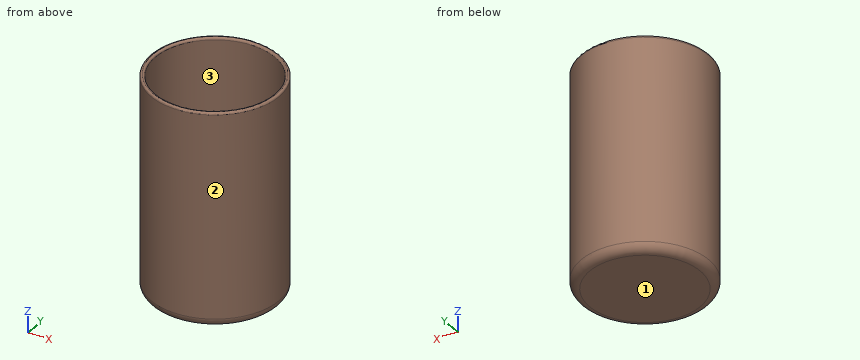
```python
from build123d import *

# Parameters (mm, degrees)
F0_R     = 38.1
F0_R_2   = 35.56
F1_DEPTH = 127
F2_R     = 38.1
F3_DEPTH = 25.4
F4_R     = 1.26999
F5_R     = 5.08
F6_R     = 5.08


# Not quite as in the source:
# - a fillet or chamfer is up to 0.001 mm smaller than in the source, because OpenCascade refuses the exact size


with BuildPart() as f1:
    # F0 (on Top) → F1 (new body)
    with BuildSketch(Plane.XY):
        Circle(F0_R)
        Circle(F0_R_2, mode=Mode.SUBTRACT)
    extrude(amount=F1_DEPTH)

    # F2 (on Top) → F3 (join)
    with BuildSketch(Plane.XY):
        Circle(F2_R)
    extrude(amount=F3_DEPTH)

    # F4 (radius 1.27 in the source; OpenCascade refuses exactly that, so slightly less here)
    f4_edges = [f1.edges().sort_by_distance(p)[0] for p in [
        (-38.1, 0, 127),
        (-35.56, 0, 127),
    ]]
    fillet(f4_edges, radius=F4_R)

    # F5
    f5_edges = [f1.edges().sort_by_distance(p)[0] for p in [
        (-38.1, 0, 0),
    ]]
    fillet(f5_edges, radius=F5_R)

    # F6
    f6_edges = [f1.edges().sort_by_distance(p)[0] for p in [
        (-35.56, 0, 25.4),
    ]]
    fillet(f6_edges, radius=F6_R)


solid = f1.part
```
Could you check a few things on this model? Use its own coordinates, in mm. Face numbers are marked on the shaded views. Coordinates: 2 decimals unless noted, no trailing zeros. Write each loop counter-clockwise with the first axis right and the second up, starting at its lowest first coordinate (ties: lowest second). Pieces come first, ordered by that corner, then holes. Notation, with made-up numbers: (-3.75, 37.25) - (30.25, 37.25) arc R12 ccw to (30.25, 56.25) - close; hole circle Ø10 at (60, 61). An arc over 180 degrees is marked (long way). Use a Markdown table: item, result.
Q1. Please list where these lines run through material, in increasing order: L1, parallel to Y at x = 0, z = 65; L2, parallel to Z at x = 1, y = 15; L3, parallel to Y at x = 30.5, z = 77.5.
Geometry check:
| item | result |
|---|---|
| L1 | y = -38.1 to -35.56, 35.56 to 38.1 |
| L2 | z = 0 to 25.4 |
| L3 | y = -22.83 to -18.28, 18.28 to 22.83 |
Q2. Thinking about a two-plate mould opening in X: for the marked faces 1, 2 and 3, which applies, +X half, -X half, draft (parallel to the pull), parting line (faces both ways), or undercut?
Geometry check:
| item | result |
|---|---|
| face 1 | draft |
| face 2 | parting line |
| face 3 | undercut |
Q3. Imagine slicing it at D-D (z = 16). List the corners of the cut face in (x, y) for me.
Geometry check:
| item | result |
|---|---|
| outline | circle Ø76.2 at (0, 0) |
Q4. I'm going to push flat-ended pins straight in: pin 1 Ø1 at (x, z) = (15, 64) entering from -Y; pin 2 Ø12 at (x, z) = (0, 80) entering from -Y; pin 3 Ø1 at (x, z) = (-10.5, 86) entering from +Y. Where does each tip first touch, or does it pass through?
Geometry check:
| item | result |
|---|---|
| pin 1 | stops at y = -35.23 |
| pin 2 | stops at y = -38.1 |
| pin 3 | stops at y = 36.76 |
Q5. Imagine slicing it at C-C (z = 66). List the corners of the cut face in (x, y) for me.
Geometry check:
| item | result |
|---|---|
| outline | circle Ø76.2 at (0, 0); hole circle Ø71.12 at (0, 0) |
